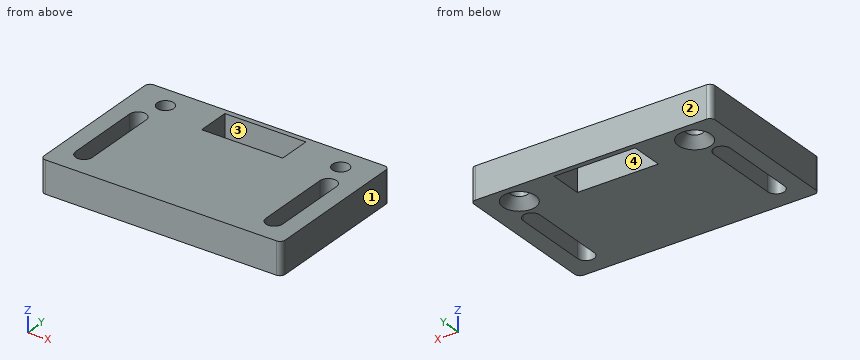
from build123d import *

# Parameters (mm, degrees)
SKETCH1_W                                        = 95
SKETCH1_H                                        = 60
BOSS_EXTRUDE1_DEPTH                              = 12.7
CSK_FOR_1_4_FLAT_HEAD_MACHINE_SCREW2_D           = 6.5278
CSK_FOR_1_4_FLAT_HEAD_MACHINE_SCREW2_CSINK_D     = 12.8778
CSK_FOR_1_4_FLAT_HEAD_MACHINE_SCREW2_CSINK_ANGLE = 82
FILLET1_R                                        = 2
FILLET2_R                                        = 2
CUT_EXTRUDE1_DEPTH                               = 78.572804513


with BuildPart() as part:
    # Sketch1 → Boss-Extrude1 (new body)
    with BuildSketch(Plane.XY):
        with Locations((0, -30)):
            Rectangle(SKETCH1_W, SKETCH1_H)
        Polygon((0, -2), (15.975, -2), (15.975, -14.9), (-15.975, -14.9), (-15.975, -2), align=None, mode=Mode.SUBTRACT)
    extrude(amount=BOSS_EXTRUDE1_DEPTH)

    # CSK for 1/4 Flat Head Machine Screw2 (through all)
    with Locations(Plane(origin=(0, 0, 0), x_dir=(-1, 0, 0), z_dir=(0, 0, -1))):
        with Locations((-34.56, -8.845086615), (34.56, -8.845086615)):
            CounterSinkHole(CSK_FOR_1_4_FLAT_HEAD_MACHINE_SCREW2_D / 2, CSK_FOR_1_4_FLAT_HEAD_MACHINE_SCREW2_CSINK_D / 2, counter_sink_angle=CSK_FOR_1_4_FLAT_HEAD_MACHINE_SCREW2_CSINK_ANGLE)

    # Fillet1
    fillet1_edges = [part.edges().sort_by_distance(p)[0] for p in [
        (-47.5, 0, 6.35),
        (-47.5, -60, 6.35),
    ]]
    fillet(fillet1_edges, radius=FILLET1_R)

    # Fillet2
    fillet2_edges = [part.edges().sort_by_distance(p)[0] for p in [
        (47.5, 0, 6.35),
        (47.5, -60, 6.35),
    ]]
    fillet(fillet2_edges, radius=FILLET2_R)

    # Sketch9 → Cut-Extrude1 (cut, through all)
    with BuildSketch(Plane(origin=(0, 0, 0), x_dir=(-1, 0, 0), z_dir=(0, 0, -1))):
        with BuildLine():
            Line((-34.215, -49.94085979), (-34.215, -19.94085979))
            ThreePointArc((-34.215, -19.94085979), (-37.515, -16.64085979), (-40.815, -19.94085979))
            Line((-40.815, -19.94085979), (-40.815, -49.94085979))
            ThreePointArc((-40.815, -49.94085979), (-37.515, -53.24085979), (-34.215, -49.94085979))
        make_face()
        with BuildLine():
            Line((40.815, -49.94085979), (40.815, -19.94085979))
            ThreePointArc((40.815, -19.94085979), (37.515, -16.64085979), (34.215, -19.94085979))
            Line((34.215, -19.94085979), (34.215, -49.94085979))
            ThreePointArc((34.215, -49.94085979), (37.515, -53.24085979), (40.815, -49.94085979))
        make_face()
    extrude(amount=-CUT_EXTRUDE1_DEPTH, mode=Mode.SUBTRACT)


solid = part.part
For this review, take the finished solid that the model builds, in its own axes (mm). Face numbers are marked on the shaded views. Give positions to 0.01 mm unless a question says otherwise; leave off trailing zeros. Order: outer loops, then holes, each group sorted by start corner. A loop starts at its lowest first (then second) coordinate and runs counter-clockwise, first axis right, second up. Notation, with made-up numbers: (39, -33) - (85, -33) arc R9 cw to (85, -20) - close; hole circle Ø11 at (26.25, 8.25). An arc over 180 degrees is marked (long way). Answer as a JSON object with one key per item and string values. Group by question number.
Item 1: Take a section at A-A on y = -21. Give the boundary of the cut face in (x, z) (3 decimals), and give its area (3 significant figures).
Item 2: Wall thickness on line 1 along X through (y, z) = (-28.5, 9) (3 decimals); line 2 along Y through (x, z) = (-34.56, 10); line 3 along X through (y, z) = (-9, 6.5) (3 decimals): over which ranges is each line inside the solid? List them lowest first.
Item 3: Draft analysis for pull direction Y (two halves, no side actions). For the marked faces 1, 2, 3 and 4, state which applies: pulls with the +Y half, pulls with the -Y half, needs draft (parallel to the pull), parting line crosses it, or undercut.
Item 4: Take a section at B-B on x = -12. Give the boundary of the cut face in (y, z), and give its area (3 significant figures).
Item 5: Take a section at C-C on z = 5.75. Give the boundary of the cut face in (x, y) (3 decimals).
Item 6: Take a section at D-D on y = -7.5. Give the number of separate pieces and of enclosed holes in the cut face, and give its area (3 significant figures).
Reported:
{
 "1": {"outline": "(-47.5, 0) - (-40.815, 0) - (-40.815, 12.7) - (-47.5, 12.7) - close; (-34.215, 0) - (34.215, 0) - (34.215, 12.7) - (-34.215, 12.7) - close; (40.815, 0) - (47.5, 0) - (47.5, 12.7) - (40.815, 12.7) - close", "area": "1,040 mm^2"},
 "2": {"line 1": "-47.5 to -40.815, -34.215 to 34.215, 40.815 to 47.5", "line 2": "-60 to -51.41, -18.47 to -12.11, -5.58 to 0", "line 3": "-47.5 to -37.82, -31.3 to -15.975, 15.975 to 31.3, 37.82 to 47.5"},
 "3": {"face 1": "needs draft", "face 2": "pulls with the +Y half", "face 3": "undercut", "face 4": "undercut"},
 "4": {"outline": "(-60, 0) - (-14.9, 0) - (-14.9, 12.7) - (-60, 12.7) - close; (-2, 0) - (0, 0) - (0, 12.7) - (-2, 12.7) - close", "area": "598 mm^2"},
 "5": {"outline": "(-47.5, -58) arc R2 ccw to (-45.5, -60) - (45.5, -60) arc R2 ccw to (47.5, -58) - (47.5, -2) arc R2 ccw to (45.5, 0) - (-45.5, 0) arc R2 ccw to (-47.5, -2) - close; hole (-40.815, -49.941) arc R3.3 ccw to (-34.215, -49.941) - (-34.215, -19.941) arc R3.3 ccw to (-40.815, -19.941) - close; hole circle Ø6.528 at (-34.56, -8.845); hole (-15.975, -14.9) - (15.975, -14.9) - (15.975, -2) - (-15.975, -2) - close; hole circle Ø6.528 at (34.56, -8.845); hole (34.215, -49.941) arc R3.3 ccw to (40.815, -49.941) - (40.815, -19.941) arc R3.3 ccw to (34.215, -19.941) - close"},
 "6": {"separate pieces": "4", "enclosed holes": "0", "area": "625 mm^2"}
}
